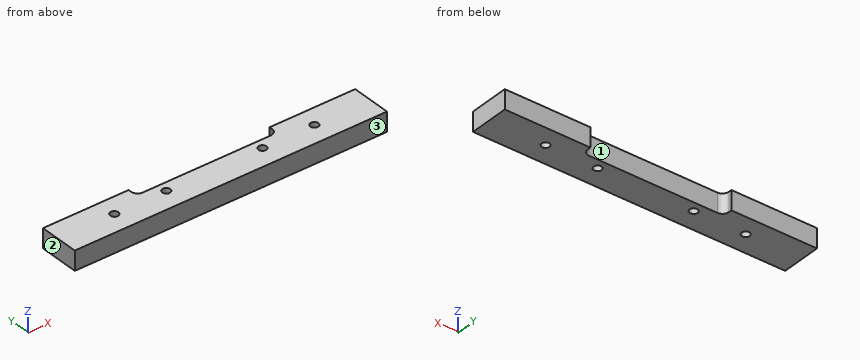
```python
from build123d import *

# Parameters (mm, degrees)
F0_R     = 2.5
F1_DEPTH = 12
F2_R     = 4


with BuildPart() as f1:
    # F0 (on Top) → F1 (new body)
    with BuildSketch(Plane.XY):
        Polygon((-97.5, -12.5), (97.5, -12.5), (97.5, 12.5), (44, 12.5), (44, 6.5), (-44, 6.5), (-44, 12.5), (-97.5, 12.5), align=None)
        with Locations((-62.5, 0.5)):
            Circle(F0_R, mode=Mode.SUBTRACT)
        with Locations((-30, 0.5)):
            Circle(F0_R, mode=Mode.SUBTRACT)
        with Locations((30, 0.5)):
            Circle(F0_R, mode=Mode.SUBTRACT)
        with Locations((62.5, 0.5)):
            Circle(F0_R, mode=Mode.SUBTRACT)
    extrude(amount=F1_DEPTH)

    # F2
    f2_edges = [f1.edges().sort_by_distance(p)[0] for p in [
        (-44, 6.5, 6),
        (44, 6.5, 6),
    ]]
    fillet(f2_edges, radius=F2_R)


solid = f1.part
```
The listing builds one solid part. Answer for the finished solid, in the listing's coordinates (mm). Face numbers are marked on the shaded views. Give positions to 0.01 mm unless a question says otherwise; leave off trailing zeros. Order: outer loops, then holes, each group sorted by start corner. A loop starts at its lowest first (then second) coordinate and runs counter-clockwise, first axis right, second up. Notation, with made-up numbers: (70, -40) - (94, -40) arc R31 cw to (94, -12) - close; hole circle Ø11 at (20.5, -3.5). An arc over 180 degrees is marked (long way). Use one line per item in the form item = value. Start each with the question number.
(1) The mould has two halves that part along X. Classify the marked faces 1, 2 and 3: released by +X, released by -X, zero draft, split by the parting line, or undercut.
(2) A cutting plane is placed at A-A, the plane y = 0.5. Write down the section's boundary in (x, z), then the cut area to 3 significant figures.
(3) A cutting plane is placed at C-C, the plane z = 2.75. Write down the section's boundary in (x, y).
(4) A cutting plane is placed at D-D, the plane x = -30. Write down the section's boundary in (y, z), then the cut area to 3 significant figures.
(5) A cutting plane is placed at B-B, the plane x = -62.5. Write down the section's boundary in (y, z).
(6) A flat-ended cylindrical pin translates along its axis: pin 1 Ø3 at (x, y) = (-30, 0.5) entering from +Z. Find the tip coordinate at first contact, or state that the pin passes through.
(7) Consider line 1 (X direction, y = 0.75, z = 9); line 2 (Y direction, x = -62.5, z = 7.5); line 3 (X direction, y = 10.75, z = 10.75). Determine where each line is inside the solid, lowest interval first. Write a range as from..to.
Ans:
q1.face_1 = undercut
q1.face_2 = released by -X
q1.face_3 = zero draft
q2.outline = (-97.5, 0) - (-65, 0) - (-65, 12) - (-97.5, 12) - close; (-60, 0) - (-32.5, 0) - (-32.5, 12) - (-60, 12) - close; (-27.5, 0) - (27.5, 0) - (27.5, 12) - (-27.5, 12) - close; (32.5, 0) - (60, 0) - (60, 12) - (32.5, 12) - close; (65, 0) - (97.5, 0) - (97.5, 12) - (65, 12) - close
q2.area = 2,100 mm^2
q3.outline = (-97.5, -12.5) - (97.5, -12.5) - (97.5, 12.5) - (44, 12.5) - (44, 10.5) arc R4 cw to (40, 6.5) - (-40, 6.5) arc R4 cw to (-44, 10.5) - (-44, 12.5) - (-97.5, 12.5) - close; hole circle Ø5 at (-62.5, 0.5); hole circle Ø5 at (-30, 0.5); hole circle Ø5 at (30, 0.5); hole circle Ø5 at (62.5, 0.5)
q4.outline = (-12.5, 0) - (-2, 0) - (-2, 12) - (-12.5, 12) - close; (3, 0) - (6.5, 0) - (6.5, 12) - (3, 12) - close
q4.area = 168 mm^2
q5.outline = (-12.5, 0) - (-2, 0) - (-2, 12) - (-12.5, 12) - close; (3, 0) - (12.5, 0) - (12.5, 12) - (3, 12) - close
q6.pin_1 = through
q7.line_1 = -97.5..-64.99, -60.01..-32.49, -27.51..27.51, 32.49..60.01, 64.99..97.5
q7.line_2 = -12.5..-2, 3..12.5
q7.line_3 = -97.5..-44, 44..97.5
